Geometry: final body of the model. Coordinates: model frame, mm. Face numbers are marked on the shaded views. Give positions to 0.01 mm unless a question says otherwise; leave off trailing zeros. Order: outer loops, then holes, each group sorted by start corner. A loop starts at its lowest first (then second) coordinate and runs counter-clockwise, first axis right, second up. Notation, with made-up numbers: (49, 14) - (81, 14) arc R18 cw to (81, 26) - close; hole circle Ø11 at (12.5, 88). An arc over 180 degrees is marked (long way). One line per item, written item: value.
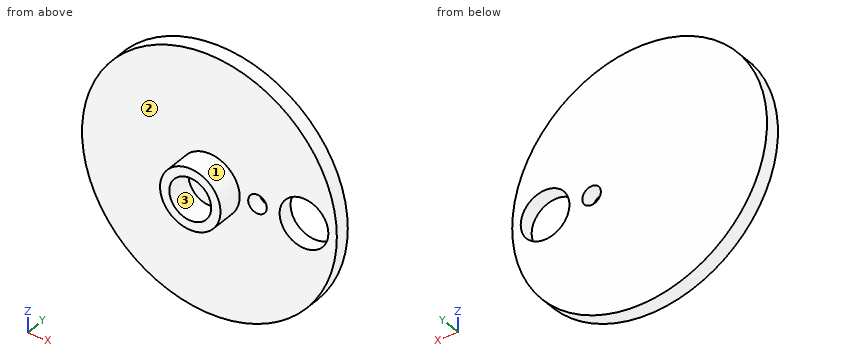
```python
from build123d import *

# Parameters (mm, degrees)
SKETCH1_R           = 4.1275
SKETCH1_R_2         = 2.8575
BOSS_EXTRUDE1_DEPTH = 3.6068
SKETCH3_R           = 17.399
SKETCH3_R_2         = 3.3274
SKETCH3_R_3         = 1.27
BOSS_EXTRUDE2_DEPTH = 2.0574


with BuildPart() as part:
    # Sketch1 → Boss-Extrude1 (new body)
    with BuildSketch(Plane(origin=(0, 0, 0), x_dir=(1, 0, 0), z_dir=(0, 1, 0))):
        Circle(SKETCH1_R)
        Circle(SKETCH1_R_2, mode=Mode.SUBTRACT)
    extrude(amount=BOSS_EXTRUDE1_DEPTH)

    # Sketch3 → Boss-Extrude2 (add)
    with BuildSketch(Plane(origin=(0, 3.6068, 0), x_dir=(1, 0, 0), z_dir=(0, 1, 0))):
        Circle(SKETCH3_R)
        with Locations((12.90955, 0)):
            Circle(SKETCH3_R_2, mode=Mode.SUBTRACT)
        with Locations((6.55955, 0)):
            Circle(SKETCH3_R_3, mode=Mode.SUBTRACT)
    extrude(amount=BOSS_EXTRUDE2_DEPTH)


solid = part.part
```
1) First-contact query: pin 1 (2 mm diameter, centred on x = -5, z = 0, fed in from -Y); pin 2 (4 mm diameter, centred on x = 9, z = -12.5, fed in from -Y); pin 3 (1 mm diameter, centred on x = 7.5, y = 1.5, fed in from -Z). Flat tips, straight axial feed; report the tip coordinate or a pass-through.
Answers below:
pin 1: y = 0
pin 2: y = 3.61
pin 3: through
2) Section A-A, the plane z = 0. Return loops of the section in (x, y).
Answers below:
outline: (-17.4, 3.61) - (-4.13, 3.61) - (-4.13, 0) - (-2.86, 0) - (-2.86, 3.61) - (2.86, 3.61) - (2.86, 0) - (4.13, 0) - (4.13, 3.61) - (5.29, 3.61) - (5.29, 5.66) - (-17.4, 5.66) - close; (7.83, 3.61) - (9.58, 3.61) - (9.58, 5.66) - (7.83, 5.66) - close; (16.24, 3.61) - (17.4, 3.61) - (17.4, 5.66) - (16.24, 5.66) - close
3) Mould query, pull axis Z, two halves, no side actions, for the marked faces 1, 2 and 3. Classes: released by +Z, released by -Z, zero draft, split by the parting line, or undercut.
Answers below:
face 1: split by the parting line
face 2: zero draft
face 3: undercut
4) Section B-B, the plane x = 7. Return loops of the section in (y, z), then the cut area to 3 significant figures.
Answers below:
outline: (3.61, -15.93) - (5.66, -15.93) - (5.66, -1.19) - (3.61, -1.19) - close; (3.61, 1.19) - (5.66, 1.19) - (5.66, 15.93) - (3.61, 15.93) - close
area: 60.6 mm^2
5) Section D-D, the plane x = 0. Return loops of the section in (y, z).
Answers below:
outline: (0, -4.13) - (3.61, -4.13) - (3.61, -17.4) - (5.66, -17.4) - (5.66, 17.4) - (3.61, 17.4) - (3.61, 4.13) - (0, 4.13) - (0, 2.86) - (3.61, 2.86) - (3.61, -2.86) - (0, -2.86) - close
6) Section C-C, the plane y = 2.2. Return loops of the section in (x, z) (1 decimal).
Answers below:
outline: circle Ø8.3 at (0, 0); hole circle Ø5.7 at (0, 0)
7) Material intervals for line 1 along X through (y, z) = (4.4, 0); line 2 along Z through (x, y) = (0, 1.3), sorted ascending.
Answers below:
line 1: -17.4 to 5.29, 7.83 to 9.58, 16.24 to 17.4
line 2: -4.13 to -2.86, 2.86 to 4.13
